from build123d import *

# Parameters (mm, degrees)
CROQUIS1_R                 = 14
SALIENTE_EXTRUIR1_DEPTH    = 200
CORTAR_EXTRUIR1_DEPTH      = 201.977610693
CORTAR_EXTRUIR1_DEPTH_BACK = 201.977610693
CROQUIS2_R                 = 13
CROQUIS3_W                 = 8
CROQUIS3_H                 = 1.4
SALIENTE_EXTRUIR2_DEPTH    = 5
EXTRUIR_L_MINA2_DEPTH      = 5
CROQUIS6_W                 = 5
CROQUIS6_H                 = 5
SALIENTE_EXTRUIR3_DEPTH    = 1
REDONDEO1_R                = 1
MATRIZL2_COUNT             = 2
MATRIZL2_PITCH             = 50
REDONDEO1_OF_MATRIZL2_R    = 1
CROQUIS8_R                 = 13.5
CORTAR_EXTRUIR2_DEPTH      = 50


with BuildPart() as part:
    # Croquis1 → Saliente-Extruir1 (new body)
    with BuildSketch(Plane.XY):
        Circle(CROQUIS1_R)
    extrude(amount=-SALIENTE_EXTRUIR1_DEPTH)

    # Croquis2 → Cortar-Extruir1 (cut, two sides: drawn at the far end of the back side and taken through both)
    with BuildSketch(Plane.XY.offset(-CORTAR_EXTRUIR1_DEPTH_BACK)):
        Circle(CROQUIS2_R)
    extrude(amount=CORTAR_EXTRUIR1_DEPTH + CORTAR_EXTRUIR1_DEPTH_BACK, mode=Mode.SUBTRACT)

    # Croquis3 → Saliente-Extruir2 (add)
    with BuildSketch(Plane.XY.offset(-100)):
        with Locations((0, 14)):
            Rectangle(CROQUIS3_W, CROQUIS3_H)
    saliente_extruir2 = extrude(amount=-SALIENTE_EXTRUIR2_DEPTH)

    # Croquis5 → Extruir-Lámina2 (add)
    with BuildSketch(Plane.XY.offset(-100)):
        with BuildLine():
            Line((-3.5, 16.142129337), (-3.5, 15.7))
            Line((-3.5, 15.7), (-3.5, 13.7))
            Line((-3.5, 13.7), (3.5, 13.7))
            Line((3.5, 13.7), (3.5, 16.142129337))
            ThreePointArc((3.5, 16.142129337), (0, 19.642129337), (-3.5, 16.142129337))
        make_face()
        with BuildLine():
            Line((-2.5, 16.142129337), (-2.5, 15.7))
            Line((-2.5, 15.7), (-2.5, 14.7))
            Line((-2.5, 14.7), (2.5, 14.7))
            Line((2.5, 14.7), (2.5, 16.142129337))
            ThreePointArc((2.5, 16.142129337), (0, 18.642129337), (-2.5, 16.142129337))
        make_face(mode=Mode.SUBTRACT)
    extruir_l_mina2 = extrude(amount=-EXTRUIR_L_MINA2_DEPTH)

    # Croquis6 → Saliente-Extruir3 (add)
    with BuildSketch(Plane(origin=(0, 14.7, 0), x_dir=(1, 0, 0), z_dir=(0, 1, 0))):
        with Locations((0, 102.5)):
            Rectangle(CROQUIS6_W, CROQUIS6_H)
    saliente_extruir3 = extrude(amount=SALIENTE_EXTRUIR3_DEPTH)

    # Redondeo1
    redondeo1_edges = [part.edges().sort_by_distance(p)[0] for p in [
        (-2.5, 15.921064668, -100),
        (0, 18.642129337, -100),
        (0, 18.642129337, -105),
        (-2.5, 15.921064668, -105),
        (2.5, 15.921064668, -105),
        (2.5, 15.921064668, -100),
        (0, 15.7, -105),
        (0, 15.7, -100),
    ]]
    fillet(redondeo1_edges, radius=REDONDEO1_R - 0.0001)  # a hair under: the kernel refuses the full size

    # MatrizL2: Saliente-Extruir2, Extruir-Lámina2, Saliente-Extruir3 ×2
    with Locations(*[(0, 0, -i * MATRIZL2_PITCH) for i in range(1, MATRIZL2_COUNT)]):
        add(saliente_extruir2)
        add(extruir_l_mina2)
        add(saliente_extruir3)

    # Redondeo1 of MatrizL2
    redondeo1_of_matrizl2_edges = [part.edges().sort_by_distance(p)[0] for p in [
        (-2.5, 15.921064668, -150),
        (0, 18.642129337, -150),
        (0, 18.642129337, -155),
        (-2.5, 15.921064668, -155),
        (2.5, 15.921064668, -155),
        (2.5, 15.921064668, -150),
        (0, 15.7, -155),
        (0, 15.7, -150),
    ]]
    fillet(redondeo1_of_matrizl2_edges, radius=REDONDEO1_OF_MATRIZL2_R - 0.0001)  # a hair under: the kernel refuses the full size

    # Croquis8 → Cortar-Extruir2 (cut)
    with BuildSketch(Plane(origin=(0, 0, -200), x_dir=(-1, 0, 0), z_dir=(0, 0, -1))):
        Circle(CROQUIS8_R)
    extrude(amount=-CORTAR_EXTRUIR2_DEPTH, mode=Mode.SUBTRACT)


solid = part.part
Input: part model. Units: mm. Frame: model coordinates. A direction names the side the tool comes from. Coordinates: 2 decimals unless noted, no trailing zeros. Order: outer loops, then holes, each group sorted by start corner. A loop starts at its lowest first (then second) coordinate and runs counter-clockwise, first axis right, second up.
1. Access query for faces 5 (the flat face through (0, 14.2, -155)), 6 (the flat face through (0, 14.2, -100)), 7 (the cylindrical face through (2.93, -13.18, -175.35)), 8 (the flat face through (0, 14.2, -105)). Directions: +Z, -Z, +X, -X, +Y, -Y. A direction counts if a zero-diameter tool reaches every point of the face in a straight line with its end or side. Return the directions, or none.
Checked values:
face 5: -Z, +Y
face 6: +Z, +Y
face 7: -Z
face 8: +Y
2. Cut plane A-A, the plane y = 0. Return loops of the section in (x, z).
Checked values:
outline: (-14, -200) - (-13.5, -200) - (-13.5, -150) - (-13, -150) - (-13, 0) - (-14, 0) - close; (13, -150) - (13.5, -150) - (13.5, -200) - (14, -200) - (14, 0) - (13, 0) - close
3. Cut plane B-B, the plane x = 11.25. Return loops of the section in (y, z), plus the area to 3 significant figures.
Checked values:
outline: (-8.33, -200) - (-7.46, -200) - (-7.46, -150) - (-6.51, -150) - (-6.51, 0) - (-8.33, 0) - close; (6.51, -150) - (7.46, -150) - (7.46, -200) - (8.33, -200) - (8.33, 0) - (6.51, 0) - close
area: 633 mm2
4. Ray query, line 1 along Y through (x, z) = (0, -167); line 2 along Y through (x, z) = (0, -35.5); line 3 along Y through (x, z) = (0, -100.5). Return the intervals inside material, ascending.
Checked values:
line 1: y = -14 to -13.5, 13.5 to 14
line 2: y = -14 to -13, 13 to 14
line 3: y = -14 to -13, 13 to 15.57, 18.78 to 19.64
5. Draft query along Y for faces 1 (the cylindrical face through (0.08, 19.64, -102.46)), 2 (the flat face through (7.1, 11.1, -150)), 3 (the cylindrical face through (12.932, -5.362, -98.6)), 4 (the flat face through (0, 14.2, -150)). Return one class per face: +Y half, -Y half, draft (parallel to the pull), parting line (faces both ways), or undercut.
Checked values:
face 1: +Y half
face 2: undercut
face 3: parting line
face 4: draft
6. Contact query for flat-ended pins moving along their axis: P1, Ø16, axis at x = 0, y = 0, coming from the +Z side; P2, Ø1.5, axis at x = 0.5, z = -102, coming from the +Y side; P3, Ø4, axis at x = 9, z = -103, coming from the +Y side; P4, Ø3, axis at x = -9, z = -147.5, coming from the +Y side. Output: stop coordinate, or through.
Checked values:
P1: passes through
P2: stops at y = 19.64
P3: stops at y = 12.12
P4: stops at y = 11.82
7. Cut plane C-C, the plane z = -158. Return loops of the section in (x, y), plus the area to 3 significant figures.
Checked values:
outline: circle Ø28 at (0, 0); hole circle Ø27 at (0, 0)
area: 43.2 mm2
8. Cut plane D-D, the plane x = 0. Count the separate pieces of the cut face and the enclosed holes in it, plus the area to 3 significant figures.
Checked values:
separate pieces: 4
enclosed holes: 0
area: 375 mm2
